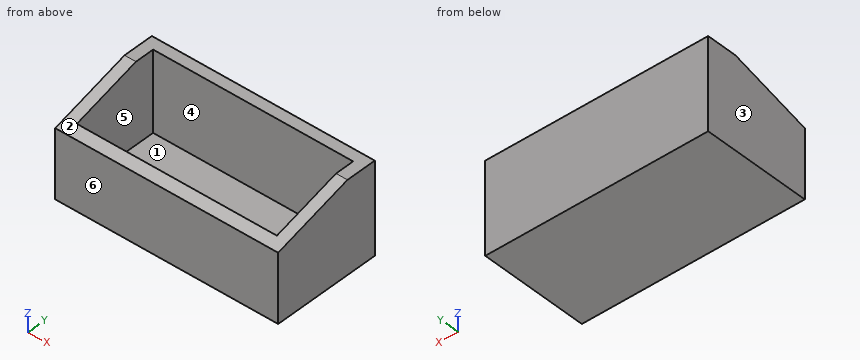
```python
from build123d import *

# Parameters (mm, degrees)
F0_W     = 495.524884
F0_H     = 203.211292
F1_DEPTH = 241.3
F2_T     = -25.4
F4_DEPTH = 495.554


with BuildPart() as f1:
    # F0 (on Front) → F1 (new body)
    with BuildSketch(Plane.XZ):
        Rectangle(F0_W, F0_H)
    extrude(amount=F1_DEPTH)

    # F2
    f2_openings = [f1.faces().sort_by_distance(p)[0] for p in [
        (0, -120.65, 101.605646),
    ]]
    offset(amount=F2_T, openings=f2_openings)

    # F3 (on face) → F4 (cut)
    with BuildSketch(Plane.YZ.offset(247.762442)):
        Polygon((-68.14377, 101.605646), (-241.3, 101.605646), (-241.3, 50.465446), align=None)
    extrude(amount=-F4_DEPTH, mode=Mode.SUBTRACT)


solid = f1.part
```
Build history of the part. All positions in model axes, mm. Face numbers are marked on the shaded views. A direction names the side the tool comes from. Coordinates: 2 decimals unless noted, no trailing zeros. Order: outer loops, then holes, each group sorted by start corner. A loop starts at its lowest first (then second) coordinate and runs counter-clockwise, first axis right, second up. Notation, with made-up numbers: M -14,2 L 10,2 A29 cw 10,41 Z; hole C 55.5,-4 d9. An arc over 180 degrees is marked long. One line per question, with ' | ' between items. Start each with the question number.
1. Cut at C-C (x = 111). Write the cut outline in (y, z).
2. Tool access for the marked faces 1 and 2: list every direction of +Z, -Z, +X, -X, +Y, -Y with a clear straight run to the whole face (end or side of a thin tool).
3. Flat gauge pins, fed straight in: P1, Ø3, axis at x = -63, y = -32, coming from the +Z side; P2, Ø2, axis at x = -129.5, z = -47.5, coming from the +Y side. Where does each tip first touch, or does it go through?
4. Cut at A-A (z = -44). Write the cut outline in (x, y), plus the area to 4 significant figures.
5. Mould opens along X. For the marked faces 3, 4, 5 and 6 say: +X half, -X half, draft (parallel to the pull), parting line (faces both ways), or undercut.
6. Wall check: line 1 along Y through (x, z) = (159, -63); line 2 along X through (y, z) = (-62, 30.5); line 3 along Y through (x, z) = (183, 69.5). Give the ranges that are in metal, low to high. Write a range as [from, to].
7. Cut at B-B (y = -50). Write the cut outline in (x, z).
The answers:
1) outline: M -241.3,-101.61 L 0,-101.61 L 0,101.61 L -25.4,101.61 L -25.4,-76.21 L -215.9,-76.21 L -215.9,57.97 L -241.3,50.47 Z
2) face 1: +Z | face 2: +Z, +X, -X, -Y
3) P1: stops at z = -76.21 | P2: stops at y = 0
4) outline: M -247.76,-241.3 L 247.76,-241.3 L 247.76,0 L -247.76,0 Z; hole M -222.36,-215.9 L 222.36,-215.9 L 222.36,-25.4 L -222.36,-25.4 Z | area: 34,850 mm2
5) face 3: -X half | face 4: undercut | face 5: undercut | face 6: draft
6) line 1: y = [-241.3, -215.9], [-25.4, 0] | line 2: x = [-247.76, -222.36], [222.36, 247.76] | line 3: y = [-25.4, 0]
7) outline: M -247.76,-101.61 L 247.76,-101.61 L 247.76,101.61 L 222.36,101.61 L 222.36,-76.21 L -222.36,-76.21 L -222.36,101.61 L -247.76,101.61 Z
